The model under review builds one solid part; all positions refer to its coordinate system, in mm. Face numbers are marked on the shaded views. A direction names the side the tool comes from. Coordinates: 2 decimals unless noted, no trailing zeros. Loops run counter-clockwise (first coordinate to the right, second up) from the corner with the lowest first, then second, coordinate; pieces in that order, holes last. Notation, with made-up numbers: (-39, -18) - (7, -18) arc R11 ccw to (7, 2) - close; hole circle Ø11 at (56, 63.25). An arc over 180 degrees is marked (long way). One line per item, written item: value. Start each with the question number.
1. We need section D-D, the plane y = 10. Give the boundary of the cut face in (x, z), then the cut area to 3 significant figures.
2. Mouldability with a two-part tool opening along Y and no side actions: class the marked faces 1, 2, 3 and 4 as +Y half, -Y half, draft (parallel to the pull), parting line (faces both ways), or undercut.
3. We need section A-A, the plane x = 27.5. Give the boundary of the cut face in (y, z), then the cut area to 3 significant figures.
4. We need section C-C, the plane x = 34.4. Give the boundary of the cut face in (y, z), then the cut area to 3 significant figures.
5. To check wall thickness, follow line 1 (Y direction, x = 4.5, z = 62.2); line 2 (X direction, y = 18, z = 74); line 3 (Z direction, x = 29.5, y = 17). State the ranges of each line that lie inside material, in increasing order.
6. For the marked faces 5, 6 and 7, list the 3-axis set-ups (+Z, -Z, +X, -X, +Y, -Y) from which the entire face can be reached by the end or side of a thin tool; tool diameter is ignored.
7. Insertion check: P1, Ø1, axis at x = 29.5, y = 11.5, coming from the -Z side; P2, Ø3, axis at y = 10, z = 62.2, coming from the -X side. Each pin has a flat end and moves straight along its axis. Give the tip position at first contact, or say it passes through.
8. We need section B-B, the plane z = 55.5. Give the boundary of the cut face in (x, y), then the cut area to 3 significant figures.
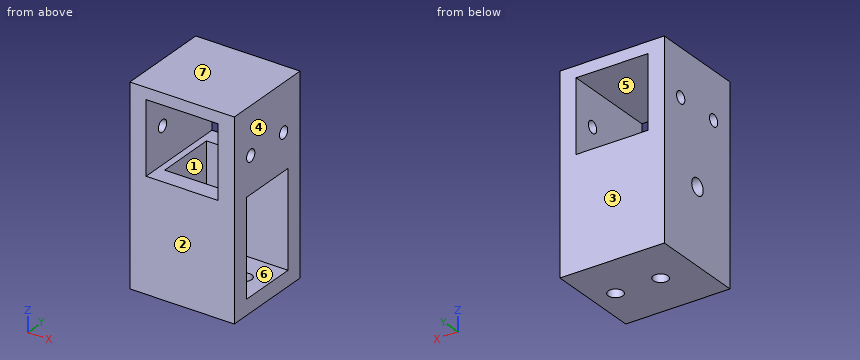
Autodesk Inventor part; units mm, degrees
ref_plane "YZ Plane" through (0, 0, 0) normal (1, 0, 0) x (0, 1, 0)
ref_plane "XZ Plane" through (0, 0, 0) normal (0, 1, 0) x (-1, 0, 0)
ref_plane "XY Plane" through (0, 0, 0) normal (0, 0, 1) x (1, 0, 0)
sketch "Sketch1" plane through (0, 0, 0) normal (0, 0, 1) x (1, 0, 0)
  line L0 (0, 0) -> (44, 0)
  line L1 (44, 0) -> (44, 40)
  line L2 (44, 40) -> (0, 40)
  line L3 (0, 40) -> (0, 0)
  dimension "d0" = 44
  dimension "d1" = 40
extrude "Extrusion1" add sketch "Sketch1" along normal blind 82
sketch "Sketch2" plane through (0, 0, 0) normal (0, -1, 0) x (1, 0, 0)
  line L0 (6.8, 77.2) -> (37.2, 77.2)
  line L1 (37.2, 77.2) -> (37.2, 46.8)
  line L2 (37.2, 46.8) -> (6.8, 46.8)
  line L3 (6.8, 46.8) -> (6.8, 77.2)
  line L4 (0, 0) -> (0, 82)
  line L5 (0, 82) -> (44, 82)
  dimension "d4" = 30.4
  dimension "d5" = 30.4
  dimension "d6" = 6.8
  dimension "d7" = 4.8
extrude "Extrusion2" cut sketch "Sketch2" against normal blind 50
sketch "Sketch4" plane through (44, 0, 0) normal (1, 0, 0) x (0, 0, -1)
  line L0 (-6.4, 7.3) -> (-46.8, 7.3)
  line L1 (-46.8, 7.3) -> (-46.8, 32.7)
  line L2 (-46.8, 32.7) -> (-6.4, 32.7)
  line L3 (-6.4, 32.7) -> (-6.4, 7.3)
  line L4 (0, 0) -> (0, 40)
  line L5 (0, 0) -> (-82, 0)
  line L6 (-46.8, 0) -> (-46.8, 40)
  point P0 (0, 20)
  point P1 (-6.4, 20)
  dimension "d10" = 25.4
  dimension "d11" = 40.4
  dimension "d13" = 7.3
extrude "Extrusion3" cut sketch "Sketch4" against normal blind 34.4
sketch "Sketch6" plane through (44, 0, 0) normal (1, 0, 0) x (0, 0, -1)
  circle A0 centre (-62.2, 30) radius 2.5
  circle A1 centre (-62.2, 10) radius 2.5
  line L0 (0, 40) -> (-82, 40)
  line L1 (0, 0) -> (-82, 0)
  point P0 (-77.2, 40)
  dimension "d24" = 5
  dimension "d25" = 10
  dimension "d26" = 5
  dimension "d27" = 10
  dimension "d28" = 15
  dimension "d29" = 15
extrude "Extrusion5" cut sketch "Sketch6" against normal blind 50
sketch "Sketch5" plane through (0, 0, 0) normal (0, 0, -1) x (-1, 0, 0)
  circle A0 centre (-15.4, 20) radius 3.1
  circle A1 centre (-34.4, 20) radius 3.1
  line L0 (-44, 40) -> (0, 40)
  line L1 (-9.6, 7.3) -> (-9.6, 32.7)
  point P0 (0, 0)
  dimension "d16" = 6.2
  dimension "d17" = 6.2
  dimension "d18" = 20
  dimension "d19" = 20
  dimension "d20" = 5.8
  dimension "d21" = 19
extrude "Extrusion4" cut sketch "Sketch5" against normal blind 34
sketch "Sketch7" plane through (9.6, 0, 0) normal (1, 0, 0) x (0, 0, -1)
  circle A0 centre (-31.4, 19.8) radius 3.5
  line L0 (-6.4, 32.7) -> (-6.4, 7.3)
  line L1 (-6.4, 7.3) -> (-46.8, 7.3)
  point P0 (0, 0)
  dimension "d32" = 7
  dimension "d33" = 25
  dimension "d34" = 12.5
extrude "Extrusion6" cut sketch "Sketch7" against normal blind 34.4
properties part number "loacell_mount1"
Findings below:
1. outline: (0, 0) - (44, 0) - (44, 6.4) - (9.6, 6.4) - (9.6, 46.8) - (6.8, 46.8) - (6.8, 59.7) - (0, 59.7) - close; (0, 64.7) - (6.8, 64.7) - (6.8, 77.2) - (37.2, 77.2) - (37.2, 64.7) - (44, 64.7) - (44, 82) - (0, 82) - close; (37.2, 46.8) - (44, 46.8) - (44, 59.7) - (37.2, 59.7) - close
1. area: 1,230 mm2
2. face 1: undercut
2. face 2: -Y half
2. face 3: +Y half
2. face 4: draft
3. outline: (0, 0) - (40, 0) - (40, 46.8) - (32.7, 46.8) - (32.7, 6.4) - (7.3, 6.4) - (7.3, 46.8) - (0, 46.8) - close; (0, 77.2) - (40, 77.2) - (40, 82) - (0, 82) - close
3. area: 1,040 mm2
4. outline: (0, 0) - (16.9, 0) - (16.9, 6.4) - (7.3, 6.4) - (7.3, 46.8) - (0, 46.8) - close; (0, 77.2) - (40, 77.2) - (40, 82) - (0, 82) - close; (23.1, 0) - (40, 0) - (40, 46.8) - (32.7, 46.8) - (32.7, 6.4) - (23.1, 6.4) - close
4. area: 998 mm2
5. line 1: 0 to 7.5, 12.5 to 27.5, 32.5 to 40
5. line 2: 0 to 6.8, 37.2 to 44
5. line 3: 0 to 6.4, 77.2 to 82
6. face 5: +Y, -Y
6. face 6: +X
6. face 7: +Z, +X, -X, +Y, -Y
7. P1: z = 0
7. P2: through
8. outline: (0, 0) - (6.8, 0) - (6.8, 40) - (0, 40) - close; (37.2, 0) - (44, 0) - (44, 40) - (37.2, 40) - close
8. area: 544 mm2
